Read the model definition and answer for the solid it produces. Units are mm, in the model's axes. Face numbers are marked on the shaded views. A direction names the side the tool comes from. Give positions to 0.01 mm unless a question says otherwise; leave off trailing zeros. Loops run counter-clockwise (first coordinate to the right, second up) from the corner with the lowest first, then second, coordinate; pieces in that order, holes last. Notation, with made-up numbers: (9.25, -31) - (61.25, -31) arc R12 ccw to (61.25, -26) - close; hole circle Ø3 at (10, -24.75). An arc over 180 degrees is marked (long way). Put each result on its own line as item: value. Start each with the question number.
1. For a pull along X with two mould halves and no side action, classify the marked faces 1, 2 and 3 as released by +X, released by -X, zero draft, split by the parting line, or undercut.
2. A cutting plane is placed at B-B, the plane z = 9. Count the separate pieces of the cut face and the enclosed holes in it, plus the area to 3 significant figures.
3. For the marked faces 4 and 5, determine the directions among +Z, -Z, +X, -X, +Y, -Y from which every point of the face is accessible in a straight line to the end or side of a thin tool.
4. Consider L1, parallel to Y at x = 1, z = 6; L2, parallel to X at y = -6, z = 7.25; L3, parallel to X at y = -0.5, z = 2.5. Determine where each line is inside the solid, lowest interval first. Write a range as from..to.
5. A cutting plane is placed at A-A, the plane y = 4.5. Determine the outline of the cut face in (x, z).
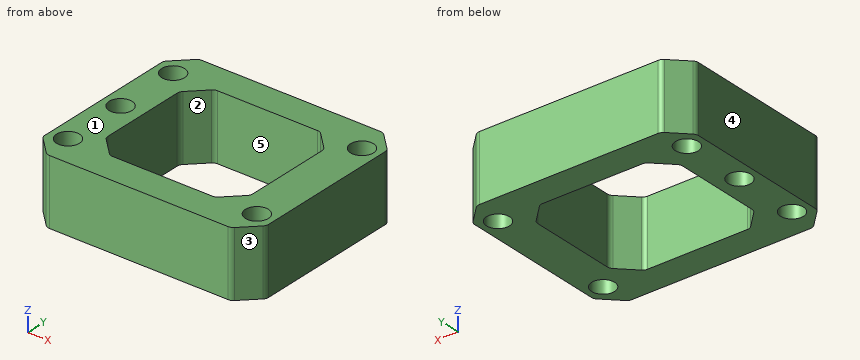
```python
from build123d import *

# Parameters (mm, degrees)
SKETCH_1_W          = 34
SKETCH_1_H          = 29
SKETCH_1_R          = 1.75
EXTRUDE_1_DEPTH     = 10
CHAMFER_1_SIZE      = 3
CUT_EXTRUDE_1_DEPTH = 11
FILLET_1_R          = 1


with BuildPart() as part:
    # 草图1 → 凸台-拉伸1 (new body)
    with BuildSketch(Plane.XY):
        Rectangle(SKETCH_1_W, SKETCH_1_H)
        with Locations((-14.35, -10)):
            Circle(SKETCH_1_R, mode=Mode.SUBTRACT)
        with Locations((-14.35, 10)):
            Circle(SKETCH_1_R, mode=Mode.SUBTRACT)
        with Locations((14.35, 10)):
            Circle(SKETCH_1_R, mode=Mode.SUBTRACT)
        with Locations((14.35, -10)):
            Circle(SKETCH_1_R, mode=Mode.SUBTRACT)
        with Locations((-14.35, 0)):
            Circle(SKETCH_1_R, mode=Mode.SUBTRACT)
    extrude(amount=EXTRUDE_1_DEPTH)

    # 倒角1
    chamfer_1_edges = [part.edges().sort_by_distance(p)[0] for p in [
        (17, -14.5, 5),
        (-17, -14.5, 5),
        (-17, 14.5, 5),
        (17, 14.5, 5),
    ]]
    chamfer(chamfer_1_edges, length=CHAMFER_1_SIZE)

    # 草图2 → 切除-拉伸1 (cut, through all)
    with BuildSketch(Plane.XY.offset(10)):
        Polygon((-11, 7), (-8, 10), (8, 10), (11, 7), (11, -7), (8, -10), (-8, -10), (-11, -7), align=None)
    extrude(amount=-CUT_EXTRUDE_1_DEPTH, mode=Mode.SUBTRACT)

    # 圆角1
    fillet_1_edges = [part.edges().sort_by_distance(p)[0] for p in [
        (17, 11.5, 5),
        (17, -11.5, 5),
        (-14, -14.5, 5),
        (14, -14.5, 5),
        (-14, 14.5, 5),
        (14, 14.5, 5),
        (-17, 11.5, 5),
        (-17, -11.5, 5),
        (-8, 10, 5),
        (8, 10, 5),
        (11, 7, 5),
        (11, -7, 5),
        (8, -10, 5),
        (-8, -10, 5),
        (-11, -7, 5),
        (-11, 7, 5),
    ]]
    fillet(fillet_1_edges, radius=FILLET_1_R)


solid = part.part
```
Return value:
1. face 1: zero draft
1. face 2: undercut
1. face 3: released by +X
2. separate pieces: 1
2. enclosed holes: 6
2. area: 498 mm2
3. face 4: +Z, -Z, -X, +Y, -Y
3. face 5: +Z, -Z
4. L1: y = -14.5..-10, 10..14.5
4. L2: x = -17..-11, 11..17
4. L3: x = -17..-16.03, -12.67..-11, 11..17
5. outline: (-17, 0) - (-11, 0) - (-11, 10) - (-17, 10) - close; (11, 0) - (17, 0) - (17, 10) - (11, 10) - close
